from build123d import *

# Parameters (mm, degrees)
SKETCH2_R           = 3.15
BOSS_EXTRUDE2_DEPTH = 3
SKETCH4_R           = 2.5
CUT_EXTRUDE1_DEPTH  = 1.5


with BuildPart() as part:
    # Sketch2 → Boss-Extrude2 (new body)
    with BuildSketch(Plane(origin=(0, 0, 0), x_dir=(1, 0, 0), z_dir=(0, 1, 0))):
        with BuildLine():
            Line((104.32233047, -139.67766953), (0, -35.355339059))
            Line((0, -35.355339059), (-104.32233047, -139.67766953))
            ThreePointArc((-104.32233047, -139.67766953), (-139.67766953, -139.67766953), (-139.67766953, -104.32233047))
            Line((-139.67766953, -104.32233047), (-35.355339059, 0))
            Line((-35.355339059, 0), (-139.67766953, 104.32233047))
            ThreePointArc((-139.67766953, 104.32233047), (-139.67766953, 139.67766953), (-104.32233047, 139.67766953))
            Line((-104.32233047, 139.67766953), (0, 35.355339059))
            Line((0, 35.355339059), (104.32233047, 139.67766953))
            ThreePointArc((104.32233047, 139.67766953), (139.67766953, 139.67766953), (139.67766953, 104.32233047))
            Line((139.67766953, 104.32233047), (35.355339059, 0))
            Line((35.355339059, 0), (139.67766953, -104.32233047))
            ThreePointArc((139.67766953, -104.32233047), (139.67766953, -139.67766953), (104.32233047, -139.67766953))
        make_face()
        with Locations((-97, 97)):
            Circle(SKETCH2_R, mode=Mode.SUBTRACT)
        with Locations((97, -97)):
            Circle(SKETCH2_R, mode=Mode.SUBTRACT)
        with Locations((97, 97)):
            Circle(SKETCH2_R, mode=Mode.SUBTRACT)
        with Locations((-97, -97)):
            Circle(SKETCH2_R, mode=Mode.SUBTRACT)
    extrude(amount=BOSS_EXTRUDE2_DEPTH)

    # Sketch4 → Cut-Extrude1 (cut)
    with BuildSketch(Plane(origin=(0, 3, 0), x_dir=(1, 0, 0), z_dir=(0, 1, 0))):
        with Locations((0, 17.67766953)):
            Circle(SKETCH4_R)
        with Locations((0, -17.67766953)):
            Circle(SKETCH4_R)
    extrude(amount=-CUT_EXTRUDE1_DEPTH, mode=Mode.SUBTRACT)


solid = part.part
Build history of the part. All positions in model axes, mm. A direction names the side the tool comes from. Round coordinates to 2 decimals unless told otherwise and drop trailing zeros. Loops run counter-clockwise (first coordinate to the right, second up) from the corner with the lowest first, then second, coordinate; pieces in that order, holes last. Notation, with made-up numbers: (-6, -5.75) -> (29, -5.75) arc R13 cw to (29, 2.25) -> close; hole circle Ø5 at (66.5, -22.5). An arc over 180 degrees is marked (long way). One line per item, written item: value. Start each with the question number.
Q1. Probe line 1 along Z through (x, y) = (0, 2.1); line 2 along X through (y, z) = (1.8, 97); line 3 along X through (y, z) = (1.5, 99). List the from-to ranges inside material, lowest first.
Q2. Cut at C-C on z = 110. List the corners of the cut face in (x, y), plus the area to 3 significant figures.
Q3. Cut at A-A on x = -122. List the corners of the cut face in (y, z).
Q4. 3-axis set-ups, long thin cutter, end or side, ignore diameter. For faces 5 (the face through (52.891, 1.479, 88.247)), 6 (the face through (-88.247, 1.479, 52.891)), 7 (the face through (88.247, 1.479, -52.891)): which of +Z, -Z, +X, -X, +Y, -Y reach the whole face in a straight line?
Q5. Two-plate mould, pull along Z, no slides. Class faces 1 (the face through (140.062, 1.479, 139.285)), 2 (the face through (2, 0, -2)), 3 (the face through (51.431, 1.479, -86.786)), 4 (the face through (-51.431, 1.479, 86.786)): released by +Z, released by -Z, zero draft, split by the parting line, or undercut.
Q6. Cut at B-B on y = 1. List the corners of the cut face in (x, z), plus the area to 3 significant figures.
Q7. Cut at D-D on x = -6.5. List the corners of the cut face in (y, z).
Q8. Drop flat-ended pins along their axis: pin 1 Ø4 at (x, z) = (0, -17.68) entering from +Y; pin 2 Ø1.5 at (y, z) = (1, -42.5) entering from +X; pin 3 Ø1 at (y, z) = (1, -67) entering from -X. Give the stop position or say it passes through.
Computed:
1. line 1: -35.36 to -20.18, -15.18 to 15.18, 20.18 to 35.36
1. line 2: -132.36 to -100.15, -93.85 to -61.64, 61.64 to 93.85, 100.15 to 132.36
1. line 3: -134.36 to -99.43, -94.57 to -63.64, 63.64 to 94.57, 99.43 to 134.36
2. outline: (-143.93, 0) -> (-74.64, 0) -> (-74.64, 3) -> (-143.93, 3) -> close; (74.64, 0) -> (143.93, 0) -> (143.93, 3) -> (74.64, 3) -> close
2. area: 416 mm²
3. outline: (0, -147) -> (3, -147) -> (3, -86.64) -> (0, -86.64) -> close; (0, 86.64) -> (3, 86.64) -> (3, 147) -> (0, 147) -> close
4. face 5: +Z, +Y, -Y
4. face 6: -X, +Y, -Y
4. face 7: +X, +Y, -Y
5. face 1: undercut
5. face 2: zero draft
5. face 3: released by -Z
5. face 4: released by +Z
6. outline: (-139.68, -104.32) arc R25 ccw to (-104.32, -139.68) -> (0, -35.36) -> (104.32, -139.68) arc R25 ccw to (139.68, -104.32) -> (35.36, 0) -> (139.68, 104.32) arc R25 ccw to (104.32, 139.68) -> (0, 35.36) -> (-104.32, 139.68) arc R25 ccw to (-139.68, 104.32) -> (-35.36, 0) -> close; hole circle Ø6.3 at (-97, -97); hole circle Ø6.3 at (-97, 97); hole circle Ø6.3 at (97, -97); hole circle Ø6.3 at (97, 97)
6. area: 35,800 mm²
7. outline: (0, -41.86) -> (3, -41.86) -> (3, 41.86) -> (0, 41.86) -> close
8. pin 1: y = 1.5
8. pin 2: x = 78.61
8. pin 3: x = -102.86
